Verification items for the finished model (mm, model axes). Face numbers are marked on the shaded views. A direction names the side the tool comes from. Round coordinates to 2 decimals unless told otherwise and drop trailing zeros. Loops run counter-clockwise (first coordinate to the right, second up) from the corner with the lowest first, then second, coordinate; pieces in that order, holes last.
from build123d import *

# Parameters (mm, degrees)
CROQUIS1_W               = 70
CROQUIS1_H               = 105
SALIENTE_EXTRUIR1_DEPTH  = 3
SALIENTE_EXTRUIR2_DEPTH  = 15
CROQUIS10_R              = 1.6
CROQUIS10_W              = 3
CROQUIS10_H              = 6
CROQUIS10_H_2            = 11
SALIENTE_EXTRUIR4_DEPTH  = 3
REDONDEO1_R              = 5
REDONDEO1_OF_SIMETR_A1_R = 5
CROQUIS12_W              = 5
CROQUIS12_H              = 15
SALIENTE_EXTRUIR5_DEPTH  = 6
CORTAR_EXTRUIR1_REACH    = 117.369
CROQUIS13_R              = 4
CORTAR_EXTRUIR2_REACH    = 117.369
CROQUIS14_R              = 1.6
CROQUIS16_R              = 2.5
CORTAR_EXTRUIR3_DEPTH    = 70
CROQUIS17_W              = 4
CROQUIS17_H              = 5
SALIENTE_EXTRUIR6_DEPTH  = 18
CHAFL_N1_SIZE            = 3
CHAFL_N2_SIZE            = 3


# Some blends are built 0.0001 mm under size
with BuildPart() as part:
    # Croquis1 → Saliente-Extruir1 (new body)
    with BuildSketch(Plane(origin=(0, 0, 0), x_dir=(1, 0, 0), z_dir=(0, 1, 0))):
        Rectangle(CROQUIS1_W, CROQUIS1_H)
    extrude(amount=SALIENTE_EXTRUIR1_DEPTH)

    # Croquis2 → Saliente-Extruir2 (add)
    with BuildSketch(Plane(origin=(0, 3, 0), x_dir=(1, 0, 0), z_dir=(0, 1, 0))):
        Polygon((-35, 52.5), (-30, 52.5), (-30, -47.5), (30, -47.5), (30, 52.5), (35, 52.5), (35, -52.5), (-35, -52.5), align=None)
    extrude(amount=SALIENTE_EXTRUIR2_DEPTH)

    # Croquis10 → Saliente-Extruir4 (add)
    # profile 1 of 6: a face of its own
    with BuildSketch(Plane(origin=(35, 0, 0), x_dir=(0, 0, -1), z_dir=(1, 0, 0))):
        Polygon((8.5, 29), (8.5, 18), (17.5, 18), (17.5, 29), (11.5, 29), align=None)
        with Locations((11.5, 21)):
            Circle(CROQUIS10_R, mode=Mode.SUBTRACT)
    # profile 2 of 6: a face of its own
    with BuildSketch(Plane(origin=(35, 0, 0), x_dir=(0, 0, -1), z_dir=(1, 0, 0))):
        Polygon((8.5, 18), (8.5, 12), (11.5, 12), (17.5, 12), (17.5, 18), align=None)
    # profile 3 of 6: a face of its own
    with BuildSketch(Plane(origin=(35, 0, 0), x_dir=(0, 0, -1), z_dir=(1, 0, 0))):
        with Locations((7, 15)):
            Rectangle(CROQUIS10_W, CROQUIS10_H)
    # profile 4 of 6: a face of its own
    with BuildSketch(Plane(origin=(35, 0, 0), x_dir=(0, 0, -1), z_dir=(1, 0, 0))):
        with Locations((7, 23.5)):
            Rectangle(CROQUIS10_W, CROQUIS10_H_2)
    # profile 5 of 6: a face of its own
    with BuildSketch(Plane(origin=(35, 0, 0), x_dir=(0, 0, -1), z_dir=(1, 0, 0))):
        Polygon((-40.5, 18), (-28.5, 18), (-28.5, 29), (-31.5, 29), (-34.5, 29), (-40.5, 29), align=None)
        with Locations((-34.5, 21)):
            Circle(CROQUIS10_R, mode=Mode.SUBTRACT)
    # profile 6 of 6: a face of its own
    with BuildSketch(Plane(origin=(35, 0, 0), x_dir=(0, 0, -1), z_dir=(1, 0, 0))):
        Polygon((-28.5, 12), (-28.5, 18), (-40.5, 18), (-40.5, 12), (-34.5, 12), (-31.5, 12), align=None)
    saliente_extruir4 = extrude(amount=SALIENTE_EXTRUIR4_DEPTH)

    # Redondeo1
    # the kernel refuses this fillet: 5 mm, written as the material it takes off along each edge
    with BuildSketch(Plane(origin=(38, 12, 5.956439237), x_dir=(-1, 0, 0), z_dir=(0, 0, -1))) as redondeo1_piece_1:
        with BuildLine():
            CenterArc((5, 4.582575695), REDONDEO1_R, 180, 66.421821522)
            Line((0, 4.582575695), (-0.1, 4.582575695))
            Line((-0.1, 4.582575695), (-0.1, 0))
            Line((-0.1, 0), (0, -0.1))
            ThreePointArc((0, -0.1), (1.5, -0.1), (2.96, -0.091651514))
            Line((2.96, -0.091651514), (3, 0))
        make_face()
    extrude(amount=34.912878475, mode=Mode.SUBTRACT)
    with BuildSketch(Plane(origin=(38, 12, 17.043560763), x_dir=(-1, 0, 0), z_dir=(0, 0, 1))) as redondeo1_piece_2:
        with BuildLine():
            CenterArc((5, -4.582575695), REDONDEO1_R, 113.578178478, 66.421821522)
            Line((0, -4.582575695), (-0.1, -4.582575695))
            Line((-0.1, -4.582575695), (-0.1, 0))
            Line((-0.1, 0), (0, 0.1))
            ThreePointArc((0, 0.1), (1.5, 0.1), (2.96, 0.091651514))
            Line((2.96, 0.091651514), (3, 0))
        make_face()
    extrude(amount=34.912878475, mode=Mode.SUBTRACT)

    # Simetría1: Saliente-Extruir4 across plane
    add(saliente_extruir4.mirror(Plane(origin=(0, 0, 0), x_dir=(0, 0, 1), z_dir=(1, 0, 0))))

    # Redondeo1 of Simetría1
    # the kernel refuses this fillet: 5 mm, written as the material it takes off along each edge
    with BuildSketch(Plane(origin=(-38, 12, 5.956439237), x_dir=(1, 0, 0), z_dir=(0, 0, -1))) as redondeo1_of_simetr_a1_piece_1:
        with BuildLine():
            CenterArc((5, -4.582575695), REDONDEO1_OF_SIMETR_A1_R, 113.578178478, 66.421821522)
            Line((0, -4.582575695), (-0.1, -4.582575695))
            Line((-0.1, -4.582575695), (-0.1, 0))
            Line((-0.1, 0), (0, 0.1))
            ThreePointArc((0, 0.1), (1.5, 0.1), (2.96, 0.091651514))
            Line((2.96, 0.091651514), (3, 0))
        make_face()
    extrude(amount=34.912878475, mode=Mode.SUBTRACT)
    with BuildSketch(Plane(origin=(-38, 12, 17.043560763), x_dir=(1, 0, 0), z_dir=(0, 0, 1))) as redondeo1_of_simetr_a1_piece_2:
        with BuildLine():
            CenterArc((5, 4.582575695), REDONDEO1_OF_SIMETR_A1_R, 180, 66.421821522)
            Line((0, 4.582575695), (-0.1, 4.582575695))
            Line((-0.1, 4.582575695), (-0.1, 0))
            Line((-0.1, 0), (0, -0.1))
            ThreePointArc((0, -0.1), (1.5, -0.1), (2.96, -0.091651514))
            Line((2.96, -0.091651514), (3, 0))
        make_face()
    extrude(amount=34.912878475, mode=Mode.SUBTRACT)

    # Croquis12 → Saliente-Extruir5 (add)
    with BuildSketch(Plane(origin=(-30, 0, 0), x_dir=(0, 0, -1), z_dir=(1, 0, 0))):
        with Locations((50, 10.5)):
            Rectangle(CROQUIS12_W, CROQUIS12_H)
    saliente_extruir5 = extrude(amount=SALIENTE_EXTRUIR5_DEPTH)

    # Simetría2: Saliente-Extruir5 across plane
    add(saliente_extruir5.mirror(Plane(origin=(0, 0, 0), x_dir=(0, 0, 1), z_dir=(1, 0, 0))))

    # Croquis13 → Cortar-Extruir1 (cut, up to next)
    with BuildSketch(Plane.XY.offset(52.5), mode=Mode.PRIVATE) as cortar_extruir1_sk1:
        with Locations((-20, 10.5)):
            Circle(CROQUIS13_R)
    cortar_extruir1_tool1 = extrude(cortar_extruir1_sk1.sketch, amount=-CORTAR_EXTRUIR1_REACH, mode=Mode.PRIVATE) & part.part
    # Croquis13 → Cortar-Extruir1 (cut, up to next)
    with BuildSketch(Plane.XY.offset(52.5), mode=Mode.PRIVATE) as cortar_extruir1_sk2:
        with Locations((0, 10.5)):
            Circle(CROQUIS13_R)
    cortar_extruir1_tool2 = extrude(cortar_extruir1_sk2.sketch, amount=-CORTAR_EXTRUIR1_REACH, mode=Mode.PRIVATE) & part.part
    # Croquis13 → Cortar-Extruir1 (cut, up to next)
    with BuildSketch(Plane.XY.offset(52.5), mode=Mode.PRIVATE) as cortar_extruir1_sk3:
        with Locations((20, 10.5)):
            Circle(CROQUIS13_R)
    cortar_extruir1_tool3 = extrude(cortar_extruir1_sk3.sketch, amount=-CORTAR_EXTRUIR1_REACH, mode=Mode.PRIVATE) & part.part
    add(cortar_extruir1_tool1.solids().sort_by_distance((-20, 10.5, 52.5))[0], mode=Mode.SUBTRACT)
    add(cortar_extruir1_tool2.solids().sort_by_distance((0, 10.5, 52.5))[0], mode=Mode.SUBTRACT)
    add(cortar_extruir1_tool3.solids().sort_by_distance((20, 10.5, 52.5))[0], mode=Mode.SUBTRACT)

    # Croquis14 → Cortar-Extruir2 (cut, up to next)
    with BuildSketch(Plane(origin=(0, 0, -52.5), x_dir=(-1, 0, 0), z_dir=(0, 0, -1)), mode=Mode.PRIVATE) as cortar_extruir2_sk1:
        with Locations((27.2, 14)):
            Circle(CROQUIS14_R)
    cortar_extruir2_tool1 = extrude(cortar_extruir2_sk1.sketch, amount=-CORTAR_EXTRUIR2_REACH, mode=Mode.PRIVATE) & part.part
    # Croquis14 → Cortar-Extruir2 (cut, up to next)
    with BuildSketch(Plane(origin=(0, 0, -52.5), x_dir=(-1, 0, 0), z_dir=(0, 0, -1)), mode=Mode.PRIVATE) as cortar_extruir2_sk2:
        with Locations((27.2, 8)):
            Circle(CROQUIS14_R)
    cortar_extruir2_tool2 = extrude(cortar_extruir2_sk2.sketch, amount=-CORTAR_EXTRUIR2_REACH, mode=Mode.PRIVATE) & part.part
    cortar_extruir2_1 = cortar_extruir2_tool1.solids().sort_by_distance((-27.2, 14, -52.5))[0]
    add(cortar_extruir2_1, mode=Mode.SUBTRACT)
    cortar_extruir2_2 = cortar_extruir2_tool2.solids().sort_by_distance((-27.2, 8, -52.5))[0]
    add(cortar_extruir2_2, mode=Mode.SUBTRACT)
    cortar_extruir2 = cortar_extruir2_1 + cortar_extruir2_2  # Cortar-Extruir2 as one shape, for the pattern or mirror that repeats it

    # Simetría3: Cortar-Extruir2 across plane
    add(cortar_extruir2.mirror(Plane(origin=(0, 0, 0), x_dir=(0, 0, 1), z_dir=(1, 0, 0))), mode=Mode.SUBTRACT)

    # Croquis16 → Cortar-Extruir3 (cut)
    with BuildSketch(Plane.ZY.offset(35)):
        with Locations((-25, 8)):
            Circle(CROQUIS16_R)
    extrude(amount=-CORTAR_EXTRUIR3_DEPTH, mode=Mode.SUBTRACT)

    # Croquis17 → Saliente-Extruir6 (add)
    with BuildSketch(Plane(origin=(0, 0, 0), x_dir=(1, 0, 0), z_dir=(0, 1, 0))):
        with Locations((33, 55)):
            Rectangle(CROQUIS17_W, CROQUIS17_H)
    saliente_extruir6 = extrude(amount=SALIENTE_EXTRUIR6_DEPTH)

    # Simetría4: Saliente-Extruir6 across plane
    add(saliente_extruir6.mirror(Plane(origin=(0, 0, 0), x_dir=(0, 0, 1), z_dir=(1, 0, 0))))

    # Chaflán1
    chafl_n1_edges = [part.edges().sort_by_distance(p)[0] for p in [
        (33, 0, -57.5),
        (-33, 0, -57.5),
    ]]
    chamfer(chafl_n1_edges, length=CHAFL_N1_SIZE)

    # Chaflán2
    chafl_n2_edges = [part.edges().sort_by_distance(p)[0] for p in [
        (38, 29, -11.5),
        (38, 29, 34.5),
    ]]
    chamfer(chafl_n2_edges, length=CHAFL_N2_SIZE - 0.0001)  # a hair under: the kernel refuses the full size


solid = part.part
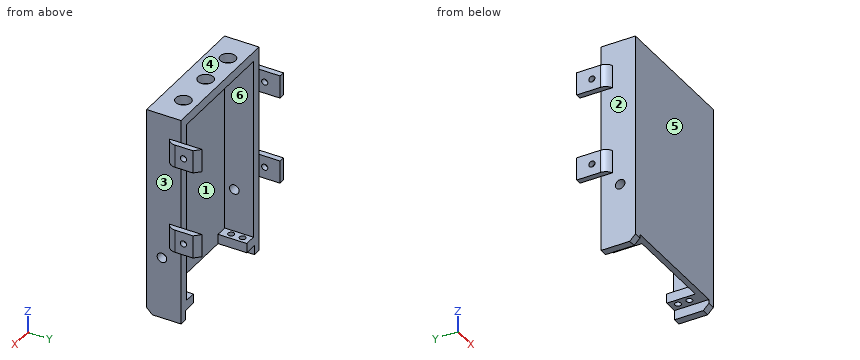
1. Tool access check on the marked faces 1, 2 and 3. Record the directions out of +Z, -Z, +X, -X, +Y, -Y that give a thin tool (end or side, any length) a straight path to the whole face; none if there is none.
2. Scan lines: L1, parallel to Y at x = -27, z = -50; L2, parallel to X at y = 17.75, z = 1; L3, parallel to Y at x = -31.4, z = -25. Record each from-to range of solid material in increasing order.
3. Section check B-B (z = 34.5). Give the number of separate pieces and of enclosed holes in the cut face, then the cut area to 3 significant figures.
4. Gauge pin test, flat ends, axial feed: P1, Ø5.5, axis at y = 7, z = -23.5, coming from the -X side; P2, Ø9, axis at y = 22, z = -10.5, coming from the +X side; P3, Ø4.5, axis at y = 12.5, z = 4.5, coming from the +X side; P4, Ø6, axis at x = 3.5, z = 4, coming from the +Y side. Record the tip position at first contact, or that the pin passes through.
5. Section check A-A (x = -20). Enter the section's corners in (y, z), then the cut area to 3 significant figures.
6. Section check D-D (z = -3). Enter the section's corners in (x, y).
7. Release check for a two-part mould opening along Z. For the marked faces 4, 5 and 6 record: released by +Z, released by -Z, zero draft, split by the parting line, or undercut.
Taken from the geometry:
1. face 1: +Y
1. face 2: -X, -Y
1. face 3: +X, -Y
2. L1: y = 0 to 6.41, 9.59 to 12.41, 15.59 to 18
2. L2: x = -35 to -30, 30 to 35
2. L3: y = 0 to 5.5, 10.5 to 18
3. separate pieces: 3
3. enclosed holes: 0
3. area: 431 mm2
4. P1: stops at x = -35
4. P2: stops at x = 38
4. P3: stops at x = 35
4. P4: stops at y = 3
5. outline: (0, -52.5) - (3, -52.5) - (3, 47.5) - (6.5, 47.5) - (6.5, 52.5) - (0, 52.5) - close; (14.5, 47.5) - (18, 47.5) - (18, 52.5) - (14.5, 52.5) - close
5. area: 350 mm2
6. outline: (-35, 0) - (35, 0) - (35, 18) - (30, 18) - (30, 3) - (-30, 3) - (-30, 18) - (-35, 18) - close
7. face 4: released by +Z
7. face 5: zero draft
7. face 6: undercut
